from build123d import *

# Parameters (mm, degrees)
SKETCH1_R           = 5
SKETCH1_R_2         = 1.5
SKETCH1_W           = 15
SKETCH1_H           = 3.175
SKETCH1_W_2         = 6.35
SKETCH1_H_2         = 16.66
BOSS_EXTRUDE1_DEPTH = 6.35


with BuildPart() as part:
    # Sketch1 → Boss-Extrude1 (new body)
    with BuildSketch(Plane.XY):
        Polygon((160, 0), (160, 18.5075), (155, 18.5075), (155, 21.6575), (160, 21.6575), (160, 38.3175), (155, 38.3175), (155, 41.4925), (160, 41.4925), (160, 60), (0, 60), (0, 41.505), (5, 41.505), (5, 38.33), (0, 38.33), (0, 21.67), (5, 21.67), (5, 18.495), (0, 18.495), (0, 0), align=None)
        with Locations((72, 30)):
            Circle(SKETCH1_R, mode=Mode.SUBTRACT)
        with Locations((98, 27)):
            Circle(SKETCH1_R_2, mode=Mode.SUBTRACT)
        with Locations((98, 33)):
            Circle(SKETCH1_R_2, mode=Mode.SUBTRACT)
        with Locations((64.5, 19.5875)):
            Rectangle(SKETCH1_W, SKETCH1_H, mode=Mode.SUBTRACT)
        with Locations((64.5, 40.4125)):
            Rectangle(SKETCH1_W, SKETCH1_H, mode=Mode.SUBTRACT)
        with Locations((22.5, 40.4125)):
            Rectangle(SKETCH1_W, SKETCH1_H, mode=Mode.SUBTRACT)
        with Locations((11.000000297, 30)):
            Rectangle(SKETCH1_W_2, SKETCH1_H_2, mode=Mode.SUBTRACT)
        with Locations((148.999999703, 29.9875)):
            Rectangle(SKETCH1_W_2, SKETCH1_H_2, mode=Mode.SUBTRACT)
        with Locations((22.5, 19.5875)):
            Rectangle(SKETCH1_W, SKETCH1_H, mode=Mode.SUBTRACT)
    extrude(amount=BOSS_EXTRUDE1_DEPTH)


solid = part.part
Can you work these out from the model? Positions are in its coordinate system, mm. A direction names the side the tool comes from. Coordinates: 2 decimals unless noted, no trailing zeros. Order: outer loops, then holes, each group sorted by start corner. A loop starts at its lowest first (then second) coordinate and runs counter-clockwise, first axis right, second up. Notation, with made-up numbers: (79.25, 86) -> (83.25, 86) arc R19 cw to (83.25, 99) -> close; hole circle Ø1 at (73.25, 12). An arc over 180 degrees is marked (long way). Use one line per item in the form item = value.
Q1. Imagine slicing it at C-C, the plane x = 24.5. List the corners of the cut face in (y, z) for me (3 decimals), then the cut area to 3 significant figures.
From the geometry:
outline = (0, 0) -> (18, 0) -> (18, 6.35) -> (0, 6.35) -> close; (21.175, 0) -> (38.825, 0) -> (38.825, 6.35) -> (21.175, 6.35) -> close; (42, 0) -> (60, 0) -> (60, 6.35) -> (42, 6.35) -> close
area = 341 mm²
Q2. Imagine slicing it at D-D, the plane z = 3. Give the number of separate pieces and of enclosed holes in the cut face, then the cut area to 3 significant figures.
From the geometry:
separate_pieces = 1
enclosed_holes = 9
area = 9,040 mm²
Q3. Imagine slicing it at B-B, the plane y = 30. List the corners of the cut face in (x, z) for me (3 decimals), then the cut area to 3 significant figures.
From the geometry:
outline = (0, 0) -> (7.825, 0) -> (7.825, 6.35) -> (0, 6.35) -> close; (14.175, 0) -> (67, 0) -> (67, 6.35) -> (14.175, 6.35) -> close; (77, 0) -> (145.825, 0) -> (145.825, 6.35) -> (77, 6.35) -> close; (152.175, 0) -> (160, 0) -> (160, 6.35) -> (152.175, 6.35) -> close
area = 872 mm²
Q4. Which directions (+Z, -Z, +X, -X, +Y, -Y) give clear straight access to the entire face, cutting with the end or side of a thin tool? Please do faces 5 (the face through (64, 38.825, 3)), 6 (the face through (158, 38.318, 3)), 7 (the face through (2, 41.505, 3)).
From the geometry:
face_5 = +Z, -Z
face_6 = +Z, -Z, +X
face_7 = +Z, -Z, -X
Q5. We'd pull the mould along X, two halves only. Please class faces 1 (the face through (15, 20, 3)), 2 (the face through (157, 41.492, 3)), 3 (the face through (160, 9, 3)), 4 (the face through (0, 30, 3)): released by +X, released by -X, zero draft, split by the parting line, or undercut.
From the geometry:
face_1 = undercut
face_2 = zero draft
face_3 = released by +X
face_4 = released by -X
Q6. Imagine slicing it at A-A, the plane x = 98. List the corners of the cut face in (y, z) for me.
From the geometry:
outline = (0, 0) -> (25.5, 0) -> (25.5, 6.35) -> (0, 6.35) -> close; (28.5, 0) -> (31.5, 0) -> (31.5, 6.35) -> (28.5, 6.35) -> close; (34.5, 0) -> (60, 0) -> (60, 6.35) -> (34.5, 6.35) -> close
Q7. I need wall thicknesses on L1, parallel to X at y = 36.5, z = 6 (3 decimals); L2, parallel to Y at x = 25.5, z = 2.75 (3 decimals); L3, parallel to Y at x = 68, z = 1.5 (3 decimals). Which ranges of each line are inside material? Lowest first, please.
From the geometry:
L1 = 0 to 7.825, 14.175 to 145.825, 152.175 to 160
L2 = 0 to 18, 21.175 to 38.825, 42 to 60
L3 = 0 to 18, 21.175 to 27, 33 to 38.825, 42 to 60
Q8. Will this pin go through, and if not, where does the flat tip stop? P1, Ø1.6, axis at y = 40.5, z = 4.5, coming from the +X side.
From the geometry:
P1 = 155
